from build123d import *

# Parameters (mm, degrees)
BOSS_EXTRU_1_DEPTH      = 580
ESQUISSE2_R             = 11.8
ENL_V_MAT_EXTRU_1_DEPTH = 10


with BuildPart() as part:
    # Esquisse1 → Boss.-Extru.1 (new body)
    with BuildSketch(Plane.XY):
        Polygon((120, 155), (10, 183), (10, 173), (120, 145), align=None)
    extrude(amount=-BOSS_EXTRU_1_DEPTH)

    # Esquisse2 → Enlèv. mat.-Extru.1 (cut)
    with BuildSketch(Plane(origin=(44.355790127, 174.254889786, 0), x_dir=(0.969097174, -0.246679281, 0), z_dir=(0.246679281, 0.969097174, 0))):
        with Locations((41.344408766, 308.745926628)):
            Circle(ESQUISSE2_R)
        with Locations((41.344408766, 270.946985721)):
            Circle(ESQUISSE2_R)
        with Locations((41.344408766, 527)):
            Circle(ESQUISSE2_R)
    extrude(amount=-ENL_V_MAT_EXTRU_1_DEPTH, mode=Mode.SUBTRACT)


solid = part.part
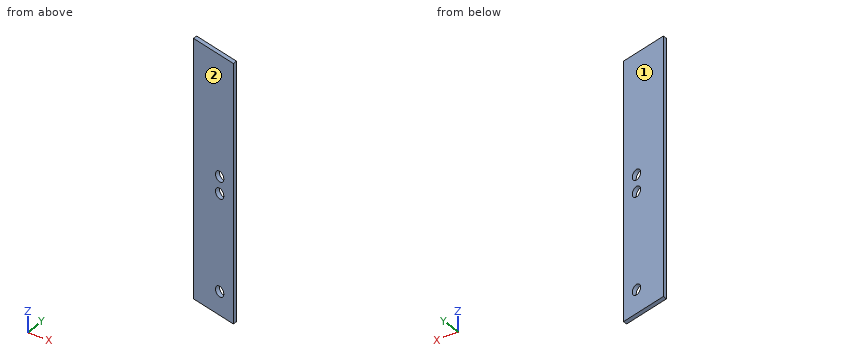
CAD build for the part. Positions are in the model's coordinates, mm. Face numbers are marked on the shaded views. Give positions to 0.01 mm unless a question says otherwise; leave off trailing zeros. Order: outer loops, then holes, each group sorted by start corner. A loop starts at its lowest first (then second) coordinate and runs counter-clockwise, first axis right, second up. Notation, with made-up numbers: (-36, -21) -> (-5, -21) arc R37 cw to (-5, 15) -> close; hole circle Ø2 at (-19, 11.5). An arc over 180 degrees is marked (long way). Return JSON: item names as keys, results as strings.
Q1. Saw through at A-A (z = -175.5). Write the cut outline in (x, y).
Working result:
{"outline": "(10, 173) -> (120, 145) -> (120, 155) -> (10, 183) -> close"}
Q2. Mould opens along Y. For the marked faces 1 and 2 say: pulls with the +Y half, pulls with the -Y half, needs draft (parallel to the pull), parting line crosses it, or undercut.
Working result:
{"face 1": "pulls with the +Y half", "face 2": "pulls with the -Y half"}
Q3. Saw through at B-B (x = 84). Count the separate pieces of the cut face and the enclosed holes in it, then the cut area to 3 significant figures.
Working result:
{"separate pieces": "4", "enclosed holes": "0", "area": "5,090 mm²"}
Q4. Drill centre lines: line 1 (Z direction, x = 85, y = 162); line 2 (Z direction, x = 80, y = 158); line 3 (Y direction, x = 19, z = -44.5). Where is each one in solid material? Low to high.
Working result:
{"line 1": "-580 to -538.75, -515.25 to -320.5, -296.99 to -282.7, -259.2 to 0", "line 2": "-580 to -538.46, -515.54 to -320.21, -297.28 to -282.41, -259.48 to 0", "line 3": "170.71 to 180.71"}
Q5. Flat gauge pins, fed straight in: pin 1 (5 mm diameter, centred on x = 31, z = -265.5, fed in from +Y); pin 2 (12 mm diameter, centred on x = 28.5, z = -263.5, fed in from -Y); pin 3 (1.5 mm diameter, centred on x = 31.5, z = -336.5, fed in from -Y). Where does each tip first touch, or does it go through?
Working result:
{"pin 1": "y = 178.29", "pin 2": "y = 166.76", "pin 3": "y = 167.34"}
Q6. Saw through at C-C (x = 113). Write the cut outline in (y, z).
Working result:
{"outline": "(146.78, -580) -> (156.78, -580) -> (156.78, 0) -> (146.78, 0) -> close"}
